For this review, take the finished solid that the model builds, in its own axes (mm). A direction names the side the tool comes from. Round coordinates to 2 decimals unless told otherwise and drop trailing zeros. Loops run counter-clockwise (first coordinate to the right, second up) from the corner with the lowest first, then second, coordinate; pieces in that order, holes last.
1. Consider section C-C on x = -14. State the section outline as (y, z) points, then the cut area to 3 significant figures.
2. Consider section B-B on y = 21. State the section outline as (x, z) points.
3. Draft analysis for pull direction X (two halves, no side actions). For faces 1 (the flat face through (34.665, 16.79, 9.86)), 2 (the flat face through (-47.217, 17.21, 9.86)), 3 (the flat face through (-45.97, 14.79, 9.86)), state which applies: released by +X, released by -X, zero draft, split by the parting line, or undercut.
4. Clearance check with flat-ended pins moving along their axes: pin 1 Ø10 at (y, z) = (20, 17.5) entering from -X; pin 2 Ø1 at (y, z) = (18.5, 15.5) entering from +X; pin 3 Ø3 at (x, z) = (48.65, 10) entering from -Y; pin 4 Ø5.5 at (x, z) = (51, 7.5) entering from +Y. State where each tip first meets the part, or that it passes through.
5. To check wall thickness, follow line 1 along X through (y, z) = (0.85, 10); line 2 along Y through (x, z) = (-30, 19); line 3 along X through (y, z) = (23.5, 18.25). State the ranges of each line that lie inside material, in increasing order.
6. Tool access review of faces 4 (the flat face through (52, 2, 10)), 5 (the flat face through (-64, 2, 10)), 6 (the flat face through (33.11, 15.21, 9.86)): name each direction out of +Z, -Z, +X, -X, +Y, -Y from which nothing blocks a thin tool from reaching the whole face with its end or side.
7. Consider section A-A on z = 10. State the section outline as (x, y) points, then the cut area to 3 significant figures.
from build123d import *

# Parameters (mm, degrees)
EXTRUDE_1_DEPTH     = 20
SKETCH_2_R          = 1.645091665
CUT_EXTRUDE_1_DEPTH = 20


with BuildPart() as part:
    # 草图1 → 凸台-拉伸1 (new body)
    with BuildSketch(Plane.XY):
        Polygon((-71.352101151, 0), (-51.352101151, 0), (-40.432994123, 30), (27.728791821, 30), (38.647898849, 0), (58.647898849, 0), (58.647898849, 2), (40.048313925, 2), (29.129206897, 32), (-41.8334092, 32), (-52.752516228, 2), (-71.352101151, 2), align=None)
    extrude(amount=EXTRUDE_1_DEPTH)

    # 草图2 → 切除-拉伸1 (cut)
    with BuildSketch(Plane(origin=(0, 0, 0), x_dir=(1, 0, 0), z_dir=(0, 1, 0))):
        with Locations((-61.352101151, -10)):
            Circle(SKETCH_2_R)
        with Locations(Location((48.647898849, -10, 0), (0, 0, 90))):
            Circle(SKETCH_2_R)
    extrude(amount=CUT_EXTRUDE_1_DEPTH, mode=Mode.SUBTRACT)


solid = part.part
Resolved:
1. outline: (30, 0) - (32, 0) - (32, 20) - (30, 20) - close
1. area: 40.0 mm2
2. outline: (-45.84, 0) - (-43.71, 0) - (-43.71, 20) - (-45.84, 20) - close; (31, 0) - (33.13, 0) - (33.13, 20) - (31, 20) - close
3. face 1: released by +X
3. face 2: released by -X
3. face 3: undercut
4. pin 1: stops at x = -48.02
4. pin 2: stops at x = 34.22
4. pin 3: passes through
4. pin 4: stops at y = 2
5. line 1: x = -71.35 to -63, -59.71 to -51.04, 38.34 to 47, 50.29 to 58.65
5. line 2: y = 30 to 32
5. line 3: x = -44.93 to -42.8, 30.09 to 32.22
6. face 4: +Z, -Z, +X, +Y
6. face 5: +Z, -Z, -X, +Y
6. face 6: +Z, -Z, -Y
7. outline: (-71.35, 0) - (-63, 0) - (-63, 2) - (-71.35, 2) - close; (-59.71, 0) - (-51.35, 0) - (-40.43, 30) - (27.73, 30) - (38.65, 0) - (47, 0) - (47, 2) - (40.05, 2) - (29.13, 32) - (-41.83, 32) - (-52.75, 2) - (-59.71, 2) - close; (50.29, 0) - (58.65, 0) - (58.65, 2) - (50.29, 2) - close
7. area: 331 mm2
